Source: CAD feature listing. Evaluate the final solid. Frame: model axes, mm. Face numbers are marked on the shaded views. A direction names the side the tool comes from. Give positions to 0.01 mm unless a question says otherwise; leave off trailing zeros. Loops run counter-clockwise (first coordinate to the right, second up) from the corner with the lowest first, then second, coordinate; pieces in that order, holes last. Notation, with made-up numbers: (-34, 73) -> (-14, 73) arc R36 cw to (-14, 111) -> close; hole circle Ø3 at (41.5, 6.5). An arc over 180 degrees is marked (long way). Return JSON: item names as keys, results as strings. Group by question number.
(1) Access query for the marked faces 1 and 2. Directions: +Z, -Z, +X, -X, +Y, -Y. A direction counts if a zero-diameter tool reaches every point of the face in a straight line with its end or side. Return the directions, or none.
(2) Draft query along Z for the marked faces 3, 4 and 5. Return one class per face: released by +Z, released by -Z, zero draft, split by the parting line, or undercut.
(3) Cut plane A-A on y = 15. Return loops of the section in (x, z).
(4) Pin query (flat end, axial travel): pin 1 (1 mm diameter, centred on x = 52, y = 18.5, fed in from +Z); pin 2 (14 mm diameter, centred on x = 42.5, z = -18.5, fed in from +Y); pin 3 (2 mm diameter, centred on y = 5, z = -3, fed in from +X); pin 4 (1.5 mm diameter, centred on x = 45.5, y = 9.5, fed in from +Z). Return the tip coordinate at first contact, or that it passes through.
(5) Ray query, line 1 (Y direction, x = 64.5, z = -8); line 2 (Y direction, x = 63, z = -8.5); line 3 (X direction, y = 23.5, z = -17.5). Return the intervals inside material, ascending. Write a range as from..to.
```python
from build123d import *

# Parameters (mm, degrees)
BOSS_EXTRUDE1_DEPTH = 74.5
FILLET1_R           = 7
FILLET2_R           = 2
FILLET3_R           = 1.5
FILLET4_R           = 3
SKETCH3_R           = 2
SKETCH3_R_2         = 1.7
SKETCH3_W           = 31
SKETCH3_H           = 23
CUT_EXTRUDE1_DEPTH  = 1.5
FILLET5_R           = 2
BOSS_EXTRUDE3_DEPTH = 1.5


with BuildPart() as part:
    # Sketch1 → Boss-Extrude1 (new body)
    with BuildSketch(Plane(origin=(0, 0, 0), x_dir=(0, 0, -1), z_dir=(1, 0, 0))):
        Polygon((-20.859650045, -2.828427125), (0, -2.828427125), (24.536605307, -2.828427125), (24.536605307, 0.171572875), (3, 0.171572875), (24.536605307, 21.708178182), (14.106780285, 32.138003205), (-10.429825023, 7.601397898), align=None)
        Polygon((19.339370465, 24.996224715), (18.879751058, 24.536605307), (21.708178182, 21.708178182), (0, 0), (-2.828427125, 2.828427125), (-3.288046533, 2.368807717), (-4.171930009, 3.252691193), (-3.712310601, 3.712310601), (-7.954951288, 7.954951288), (13.753226894, 29.663129471), (17.995867581, 25.420488784), (18.455486989, 25.880108191), align=None, mode=Mode.SUBTRACT)
    extrude(amount=BOSS_EXTRUDE1_DEPTH)

    # Fillet1
    fillet1_edges = [part.edges().sort_by_distance(p)[0] for p in [
        (37.25, -2.828427125, 20.859650045),
    ]]
    fillet(fillet1_edges, radius=FILLET1_R)

    # Fillet2
    fillet2_edges = [part.edges().sort_by_distance(p)[0] for p in [
        (37.25, 32.138003205, -14.106780285),
        (37.25, 21.708178182, -24.536605307),
        (37.25, 29.663129471, -13.753226894),
        (37.25, 7.954951288, 7.954951288),
        (37.25, 0, 0),
        (37.25, 21.708178182, -21.708178182),
    ]]
    fillet(fillet2_edges, radius=FILLET2_R)

    # Fillet3
    fillet3_edges = [part.edges().sort_by_distance(p)[0] for p in [
        (37.25, -2.828427125, -24.536605307),
        (37.25, 0.171572875, -24.536605307),
    ]]
    fillet(fillet3_edges, radius=FILLET3_R - 0.0001)  # a hair under: the kernel refuses the full size

    # Fillet4
    fillet4_edges = [part.edges().sort_by_distance(p)[0] for p in [
        (37.25, 0.171572875, -3),
    ]]
    fillet(fillet4_edges, radius=FILLET4_R)

    # Sketch3 → Cut-Extrude1 (cut)
    with BuildSketch(Plane(origin=(0, 9.01561146, 9.01561146), x_dir=(1, 0, 0), z_dir=(0, 0.7071067811865475, 0.7071067811865476))):
        with Locations(Location((11, 3.85, 0), (0, 0, 270))):
            Circle(SKETCH3_R)
        with Locations(Location((12.944543648, 17.405456352, 0), (0, 0, 270))):
            Circle(SKETCH3_R_2)
        with Locations(Location((12.944543648, 21.294543648, 0), (0, 0, 270))):
            Circle(SKETCH3_R_2)
        with Locations(Location((9.055456352, 21.294543648, 0), (0, 0, 270))):
            Circle(SKETCH3_R_2)
        with Locations(Location((9.055456352, 17.405456352, 0), (0, 0, 270))):
            Circle(SKETCH3_R_2)
        with Locations((34.5, 15.35)):
            Rectangle(SKETCH3_W, SKETCH3_H)
    extrude(amount=-CUT_EXTRUDE1_DEPTH, mode=Mode.SUBTRACT)

    # Fillet5
    fillet5_edges = [part.edges().sort_by_distance(p)[0] for p in [
        (19, 11.207642482, 5.762920267),
        (19, 27.471098449, -10.500535701),
        (50, 27.471098449, -10.500535701),
        (50, 11.207642482, 5.762920267),
    ]]
    fillet(fillet5_edges, radius=FILLET5_R)

    # Sketch4 → Boss-Extrude3 (add)
    with BuildSketch(Plane.ZY):
        with BuildLine():
            Line((-23.036605307, -2.828427125), (3.960155108, -2.828427125))
            ThreePointArc((3.960155108, -2.828427125), (10.427311836, 1.492788849), (8.909902577, 9.121320344))
            Line((8.909902577, 9.121320344), (-12.692566722, 30.723789643))
            ThreePointArc((-12.692566722, 30.723789643), (-14.106780285, 31.30957608), (-15.520993847, 30.723789643))
            Line((-15.520993847, 30.723789643), (-23.122391745, 23.122391745))
            ThreePointArc((-23.122391745, 23.122391745), (-23.708178182, 21.708178182), (-23.122391745, 20.29396462))
            Line((-23.122391745, 20.29396462), (-8.121320344, 5.292893219))
            ThreePointArc((-8.121320344, 5.292893219), (-7.47100209, 2.023522578), (-10.242640687, 0.171572875))
            Line((-10.242640687, 0.171572875), (-23.036605307, 0.171572875))
            ThreePointArc((-23.036605307, 0.171572875), (-24.097265479, -0.267766953), (-24.536605307, -1.328427125))
            ThreePointArc((-24.536605307, -1.328427125), (-24.097265479, -2.389087297), (-23.036605307, -2.828427125))
        make_face()
    extrude(amount=BOSS_EXTRUDE3_DEPTH)


solid = part.part
```
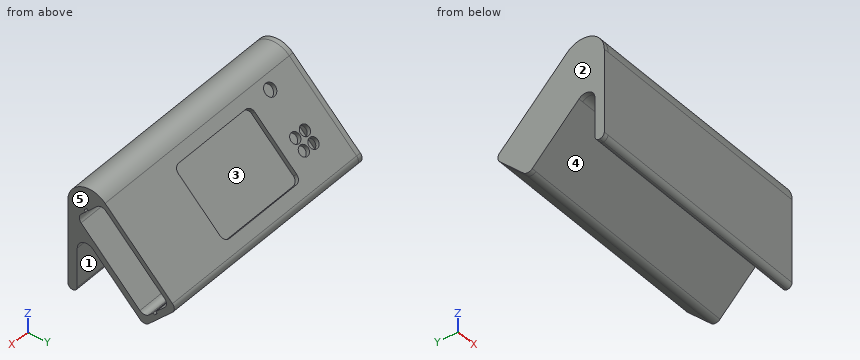
Answers:
{
 "1": {"face 1": "-Z, +X, -X", "face 2": "+Z, -Z, -X, +Y, -Y"},
 "2": {"face 3": "undercut", "face 4": "released by -Z", "face 5": "zero draft"},
 "3": {"outline": "(-1.5, -17.83) -> (74.5, -17.83) -> (74.5, -15) -> (0, -15) -> (0, 0.91) -> (19, 0.91) -> (19, 3.03) -> (-1.5, 3.03) -> close; (50, 0.91) -> (74.5, 0.91) -> (74.5, 3.03) -> (50, 3.03) -> close"},
 "4": {"pin 1": "z = 0.03", "pin 2": "y = 31.31", "pin 3": "x = 0", "pin 4": "z = 9.26"},
 "5": {"line 1": "-2.83..1.18, 5.16..8, 23.91..26.03", "line 2": "-2.83..0.73, 5.67..8.5, 24.41..26.53", "line 3": "-1.5..0"}
}
